```python
from build123d import *

# Parameters (mm, degrees)
SKETCH1_R           = 6
BOSS_EXTRUDE1_DEPTH = 7.5
SKETCH2_R           = 21.5
BOSS_EXTRUDE2_DEPTH = 3.2
SKETCH3_R           = 2
CUT_EXTRUDE1_DEPTH  = 11.7
SKETCH4_R           = 1.25
CUT_EXTRUDE2_DEPTH  = 11.7
CIRPATTERN1_COUNT   = 4
SKETCH5_R           = 3
CUT_EXTRUDE3_DEPTH  = 6.2
SKETCH6_R           = 3
CUT_EXTRUDE4_DEPTH  = 3.5


with BuildPart() as part:
    # Sketch1 → Boss-Extrude1 (new body)
    with BuildSketch(Plane(origin=(0, 0, 0), x_dir=(1, 0, 0), z_dir=(0, 1, 0))):
        Circle(SKETCH1_R)
    extrude(amount=BOSS_EXTRUDE1_DEPTH)

    # Sketch2 → Boss-Extrude2 (add)
    with BuildSketch(Plane(origin=(0, 7.5, 0), x_dir=(1, 0, 0), z_dir=(0, 1, 0))):
        Circle(SKETCH2_R)
    extrude(amount=BOSS_EXTRUDE2_DEPTH)

    # Sketch3 → Cut-Extrude1 (cut, through all)
    with BuildSketch(Plane(origin=(0, 10.7, 0), x_dir=(1, 0, 0), z_dir=(0, 1, 0))):
        with Locations((0, 16)):
            Circle(SKETCH3_R)
        with Locations((8, 16)):
            Circle(SKETCH3_R)
        with Locations((-8, 16)):
            Circle(SKETCH3_R)
    cut_extrude1 = extrude(amount=-CUT_EXTRUDE1_DEPTH, mode=Mode.SUBTRACT)

    # Sketch4 → Cut-Extrude2 (cut, through all)
    with BuildSketch(Plane(origin=(0, 10.7, 0), x_dir=(1, 0, 0), z_dir=(0, 1, 0))):
        Circle(SKETCH4_R)
    extrude(amount=-CUT_EXTRUDE2_DEPTH, mode=Mode.SUBTRACT)

    # CirPattern1: Cut-Extrude1 ×4 about axis
    cirpattern1_axis = Axis((0, 0, 0), (0, 1, 0))
    for i in range(1, CIRPATTERN1_COUNT):
        add(cut_extrude1.rotate(cirpattern1_axis, i * 360 / CIRPATTERN1_COUNT), mode=Mode.SUBTRACT)

    # Sketch5 → Cut-Extrude3 (cut)
    with BuildSketch(Plane(origin=(0, 10.7, 0), x_dir=(1, 0, 0), z_dir=(0, 1, 0))):
        Circle(SKETCH5_R)
    extrude(amount=-CUT_EXTRUDE3_DEPTH, mode=Mode.SUBTRACT)

    # Sketch6 → Cut-Extrude4 (cut)
    with BuildSketch(Plane.XZ):
        Circle(SKETCH6_R)
    extrude(amount=-CUT_EXTRUDE4_DEPTH, mode=Mode.SUBTRACT)


solid = part.part
```
Could you check a few things on this model? Use its own coordinates, in mm. A direction names the side the tool comes from. Round coordinates to 2 decimals unless told otherwise and drop trailing zeros. Loops run counter-clockwise (first coordinate to the right, second up) from the corner with the lowest first, then second, coordinate; pieces in that order, holes last. Notation, with made-up numbers: (7, -10) - (62, -10) arc R19 cw to (62, 21) - close; hole circle Ø7 at (68.5, -2.75). An arc over 180 degrees is marked (long way). Answer in a Markdown table with one row per item. Add a question column.
(1) I'm going to push flat-ended pins straight in: pin 1 (5 mm diameter, centred on x = 0, z = -16, fed in from +Y); pin 2 (2 mm diameter, centred on x = 0, z = 0, fed in from -Y); pin 3 (6 mm diameter, centred on x = 10, y = 7, fed in from +Z); pin 4 (6 mm diameter, centred on x = 14.5, z = -4, fed in from -Y). Where does each tip first touch, or does it pass through?
(2) If we section it at D-D (z = 8): Please give me the cut outline in (x, y).
(3) If we mould it in two halves opening along Z, with no side actions, what happens to faces 1 (the face through (-2.799, 9.078, -21.317)), 2 (the face through (-3, 0, 1)), 3 (the face through (1, 4.5, 1))? For each: pulls with the +Z half, pulls with the -Z half, needs draft (parallel to the pull), parting line crosses it, or undercut.
(4) For faces 4 (the face through (-6, 4, 0)), 5 (the face through (-3, 8, 0)), 6 (the face through (-18, 9, 0)), which set-ups out of +Z, -Z, +X, -X, +Y, -Y let a thin tool reach every point of the face, with its end or its side?
(5) If we section it at A-A (x = -8): Please give me the cut outline in (y, z), plus the area to 3 significant figures.
(6) If we section it at B-B (y = 9.5): State how many separate pieces and enclosed holes the cut face has, plus the area to 3 significant figures.
(7) If we section it at C-C (x = -15): Please give me the cut outline in (y, z).
(8) I need wall thicknesses on line 1 along Z through (x, y) = (0, 10); line 2 along Z through (x, y) = (0, 6.75). Which ranges of each line are inside material? Lowest first, please.
Model answer:
| question | item | result |
|---|---|---|
| 1 | pin 1 | stops at y = 10.7 |
| 1 | pin 2 | passes through |
| 1 | pin 3 | stops at z = 20.31 |
| 1 | pin 4 | stops at y = 7.5 |
| 2 | outline | (-19.96, 7.5) - (-18, 7.5) - (-18, 10.7) - (-19.96, 10.7) - close; (-14, 7.5) - (14, 7.5) - (14, 10.7) - (-14, 10.7) - close; (18, 7.5) - (19.96, 7.5) - (19.96, 10.7) - (18, 10.7) - close |
| 3 | face 1 | parting line crosses it |
| 3 | face 2 | needs draft |
| 3 | face 3 | undercut |
| 4 | face 4 | -Y |
| 4 | face 5 | +Y |
| 4 | face 6 | +Y, -Y |
| 5 | outline | (7.5, -19.96) - (10.7, -19.96) - (10.7, -18) - (7.5, -18) - close; (7.5, -14) - (10.7, -14) - (10.7, 14) - (7.5, 14) - close; (7.5, 18) - (10.7, 18) - (10.7, 19.96) - (7.5, 19.96) - close |
| 5 | area | 102 mm² |
| 6 | separate pieces | 1 |
| 6 | enclosed holes | 13 |
| 6 | area | 1,270 mm² |
| 7 | outline | (7.5, -15.4) - (10.7, -15.4) - (10.7, -9.73) - (7.5, -9.73) - close; (7.5, -6.27) - (10.7, -6.27) - (10.7, -1.73) - (7.5, -1.73) - close; (7.5, 1.73) - (10.7, 1.73) - (10.7, 6.27) - (7.5, 6.27) - close; (7.5, 9.73) - (10.7, 9.73) - (10.7, 15.4) - (7.5, 15.4) - close |
| 8 | line 1 | z = -21.5 to -18, -14 to -3, 3 to 14, 18 to 21.5 |
| 8 | line 2 | z = -6 to -3, 3 to 6 |
